```python
from build123d import *

# Parameters (mm, degrees)
F0_R     = 10.9474
F1_DEPTH = 6.35


with BuildPart() as f1:
    # F0 (on Front) → F1 (new body)
    with BuildSketch(Plane.XZ):
        with BuildLine():
            ThreePointArc((-13.2685446816, -5.0396682469), (-8.0598548082, -11.6829480217), (0, -14.1933975498))
            ThreePointArc((0, -14.1933975498), (6.7698516874, -12.4748403652), (11.90029643, -7.7353396101))
            add(Edge.make_bspline(
                [(11.90029643, -7.7353396101), (12.0535593312, -7.4829899095), (12.2107162371, -7.2236926197), (12.3714754304, -6.9569483023)],
                knots=[0.9591774425, 0.9591774425, 0.9591774425, 0.9591774425, 1, 1, 1, 1], degree=3))
            ThreePointArc((12.3714754304, -6.9569483023), (13.7303642171, -3.5957798142), (14.1933975498, 0))
            ThreePointArc((14.1933975498, 0), (0, 14.1933975498), (-14.1933975498, 0))
            ThreePointArc((-14.1933975498, 0), (-13.9602697606, -2.5619137801), (-13.2685446816, -5.0396682469))
        make_face()
        with BuildLine():
            ThreePointArc((0, -10.9474), (-7.7409807764, 7.7409807764), (10.9474, 0))
            ThreePointArc((10.9474, 0), (7.7409807764, -7.7409807764), (0, -10.9474))
        make_face(mode=Mode.SUBTRACT)
        with BuildLine():
            ThreePointArc((11.90029643, -7.7353396101), (6.7698516874, -12.4748403652), (0, -14.1933975498))
            ThreePointArc((0, -14.1933975498), (-8.0598548082, -11.6829480217), (-13.2685446816, -5.0396682469))
            add(Edge.make_bspline(
                [(-11.1718252314, -20.4150509073), (-10.2752013229, -17.9365202276), (-7.1442353987, -14.5969973645), (-11.864830176, -8.898419344), (-13.2685446816, -5.0396682469)],
                knots=[0, 0, 0, 0, 0.4355275546, 1, 1, 1, 1], degree=3))
            ThreePointArc((-11.1718252314, -20.4150509073), (-0.6968379156, -46.5203883622), (10.4937985181, -20.7137291613))
            add(Edge.make_bspline(
                [(10.4937985181, -20.7137291613), (9.1935984748, -18.2370298329), (7.5397029576, -14.7602557648), (10.0158135325, -10.8381693983), (11.90029643, -7.7353396101)],
                knots=[0, 0, 0, 0, 0.4572333258, 0.9591774425, 0.9591774425, 0.9591774425, 0.9591774425], degree=3))
        make_face()
        with BuildLine():
            ThreePointArc((10.9474, -30.3784), (-7.7409807764, -38.1193807764), (0, -19.431))
            ThreePointArc((0, -19.431), (7.7409807764, -22.6374192236), (10.9474, -30.3784))
        make_face(mode=Mode.SUBTRACT)
        with BuildLine():
            add(Edge.make_bspline(
                [(11.90029643, -7.7353396101), (12.0535593312, -7.4829899095), (12.2107162371, -7.2236926197), (12.3714754304, -6.9569483023)],
                knots=[0.9591774425, 0.9591774425, 0.9591774425, 0.9591774425, 1, 1, 1, 1], degree=3))
            ThreePointArc((11.90029643, -7.7353396101), (12.1421250434, -7.3499206416), (12.3714754304, -6.9569483023))
        make_face()
        with BuildLine():
            add(Edge.make_bspline(
                [(-14.1933975498, 0), (-14.7271984955, 6.909354162), (-8.5857084967, 14.3779721791), (-10.7006047161, 18.4330450096), (-11.7443399906, 20.6074653511)],
                knots=[0, 0, 0, 0, 0.6155147833, 1, 1, 1, 1], degree=3))
            ThreePointArc((-14.1933975498, 0), (0, 14.1933975498), (14.1933975498, 0))
            add(Edge.make_bspline(
                [(14.1933975498, 0), (14.1953765387, 8.5541345291), (8.2574436372, 15.3379896379), (9.9090943029, 17.8862823832), (10.6425855816, 19.5242241137)],
                knots=[0, 0, 0, 0, 0.6724502865, 1, 1, 1, 1], degree=3))
            ThreePointArc((10.6425855816, 19.5242241137), (0.6848487841, 45.6041133823), (-11.7443399906, 20.6074653511))
        make_face()
        with Locations((-0.0517107891, 30.3819230013)):
            Circle(F0_R, mode=Mode.SUBTRACT)
    extrude(amount=F1_DEPTH)


solid = f1.part
```
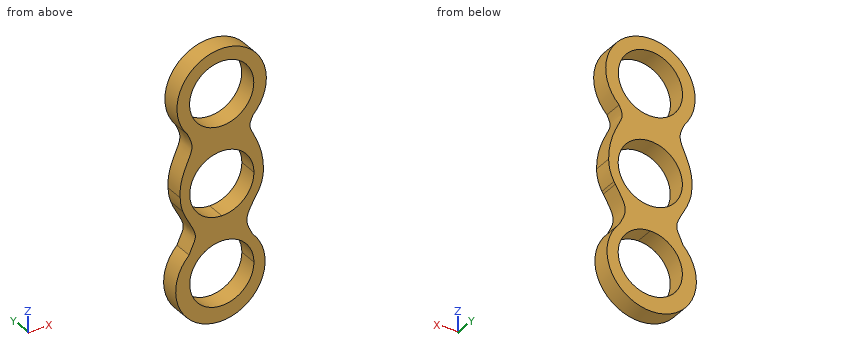
The listing builds one solid part. Answer for the finished solid, in the listing's coordinates (mm). Coordinates: 2 decimals unless noted, no trailing zeros. Write each loop counter-clockwise with the first axis right and the second up, starting at its lowest first coordinate (ties: lowest second). Pieces come first, ordered by that corner, then holes. Notation, with made-up numbers: (9, 89) -> (57, 89) arc R27 ccw to (57, 123) -> close; hole circle Ø10 at (8.25, 20). An arc over 180 degrees is marked (long way). Write each question's results on one line, items separated by ' | '. Start each with the question number.
1) A cutting plane is placed at B-B (z = -37). Determine the outline of the cut face in (x, y).
2) A cutting plane is placed at A-A (x = -7). Determine the outline of the cut face in (y, z), then the cut area to 3 significant figures.
3) Flat-ended cylindrical pins translate along their axes: pin 1 Ø1.5 at (y, z) = (-5.5, -17) entering from -X; pin 2 Ø1 at (x, z) = (8.5, -3) entering from +Y; pin 3 Ø2 at (y, z) = (-4, 28) entering from +X; pin 4 Ø2 at (x, y) = (1.5, -5) entering from -Z. Find the tip coordinate at first contact, or state that the pin passes through.
4) Straight lines are drawn through the part: probe 1 along Z at (x, y) = (3, -5.75); probe 2 along Z at (x, y) = (-3.5, -4); probe 3 along Z at (x, y) = (12, -2). For each, find the intervals that lie inside material, in ascending order.
5) A cutting plane is placed at C-C (x = 4). Determine the outline of the cut face in (y, z).
6) A cutting plane is placed at D-D (y = -5). Count the separate pieces of the cut face and the enclosed holes in it, then the cut area to 3 significant figures.
Values follow:
1) outline: (-14.61, -6.35) -> (-8.72, -6.35) -> (-8.72, 0) -> (-14.61, 0) -> close; (8.72, -6.35) -> (13.64, -6.35) -> (13.64, 0) -> (8.72, 0) -> close
2) outline: (-6.35, -45.06) -> (0, -45.06) -> (0, -38.8) -> (-6.35, -38.8) -> close; (-6.35, -21.96) -> (0, -21.96) -> (0, -8.42) -> (-6.35, -8.42) -> close; (-6.35, 8.42) -> (0, 8.42) -> (0, 21.92) -> (-6.35, 21.92) -> close; (-6.35, 38.84) -> (0, 38.84) -> (0, 43.95) -> (-6.35, 43.95) -> close | area: 244 mm²
3) pin 1: x = -9.95 | pin 2: through | pin 3: x = 15.13 | pin 4: z = -46.49
4) probe 1: -46.12 to -40.91, -19.85 to -10.53, 10.53 to 19.87, 40.9 to 45.31 | probe 2: -46.22 to -40.75, -20.01 to -10.37, 10.37 to 19.99, 40.77 to 45.23 | probe 3: -40.02 to -22.54, -7.58 to 10.4, 21.05 to 39.71
5) outline: (-6.35, -45.85) -> (0, -45.85) -> (0, -40.57) -> (-6.35, -40.57) -> close; (-6.35, -20.19) -> (0, -20.19) -> (0, -10.19) -> (-6.35, -10.19) -> close; (-6.35, 10.19) -> (0, 10.19) -> (0, 20.21) -> (-6.35, 20.21) -> close; (-6.35, 40.55) -> (0, 40.55) -> (0, 45.07) -> (-6.35, 45.07) -> close
6) separate pieces: 1 | enclosed holes: 3 | area: 1,130 mm²
